The model under review builds one solid part; all positions refer to its coordinate system, in mm. A direction names the side the tool comes from. Round coordinates to 2 decimals unless told otherwise and drop trailing zeros. Order: outer loops, then holes, each group sorted by start corner. A loop starts at its lowest first (then second) coordinate and runs counter-clockwise, first axis right, second up.
1) Machinability: for faces 5 (the face through (0.8, -1.82, -0.54)), 6 (the face through (-0.13, 7.49, 3.79)), 7 (the face through (0, 3, 7.25)), which of the approach directions +Z, -Z, +X, -X, +Y, -Y give a long, thin tool a straight path to every point of the face, cutting with its end or side? Answer none if there is none.
2) Clearance check with flat-ended pins moving along their axes: P1, Ø0.7, axis at x = 0, y = -2, coming from the -Z side; P2, Ø1, axis at x = 3.5, y = -1, coming from the +Z side; P3, Ø3, axis at y = 3.5, z = 2.5, coming from the +X side; P4, Ø0.7, axis at x = 0, y = -2.5, coming from the +Z side. State where each tip first meets the part, or that it passes through.
3) Mouldability with a two-part tool opening along Y and no side actions: class faces 1 (the face through (0, -3.7, -0.6)), 2 (the face through (0, 10.7, 0)), 3 (the face through (-0.694, 3.376, 4.046)), 4 (the face through (-0.8, -1.82, -0.56)) as pulls with the +Y half, pulls with the -Y half, needs draft (parallel to the pull), parting line crosses it, or undercut.
4) To check wall thickness, follow L1, parallel to Y at x = 0, z = 3.75; L2, parallel to Y at x = 2, z = -3.75; L3, parallel to Z at x = 2.25, y = 8. State the ranges of each line that lie inside material, in increasing order.
5) Consider section D-D (x = 1.25). Give the boundary of the cut face in (y, z), then the cut area to 3 significant figures.
6) Consider section B-B (z = 1.25). Give the boundary of the cut face in (x, y).
7) Consider section A-A (y = -1.5). Give the boundary of the cut face in (x, z), then the cut area to 3 significant figures.
8) Consider section C-C (y = 1.75). Give the boundary of the cut face in (x, z), then the cut area to 3 significant figures.
Autodesk Fusion 360 part; units mm, degrees
sketch "Sketch1" plane through (0, 0, 0) normal (0, 1, 0) x (1, 0, 0)
  line L0 (4.5, -7.25) -> (-4.5, -7.25)
  line L1 (-4.5, -7.25) -> (-4.5, 7.25)
  line L2 (-4.5, 7.25) -> (4.5, 7.25)
  line L3 (4.5, 7.25) -> (4.5, -7.25)
  line L4 (4.5, -7.25) -> (-4.5, 7.25) construction
  line L5 (-4.5, -7.25) -> (4.5, 7.25) construction
  line L6 (0, -7.25) -> (0, 7.25) construction
  circle A0 centre (4.8, 3.65) radius 0.5
  circle A1 centre (4.8, 3.05) radius 0.5
  line L7 (4.8, 3.05) -> (5.3, 3.05) construction
  line L8 (4.8, 3.65) -> (5.3, 3.65) construction
  line L9 (5.3, 3.05) -> (5.3, 3.65)
  line L10 (4.8, 3.65) -> (4.3, 3.65) construction
  line L11 (4.8, 3.05) -> (4.3, 3.05) construction
  line L12 (4.3, 3.05) -> (4.3, 3.65)
  line L13 (4.8, 3.05) -> (4.8, 3.65) construction
  line L14 (0.3, 0.05) -> (-0.3, 0.05)
  line L15 (0.3, 0.55) -> (0.3, 1.05) construction
  line L16 (0.3, 0.55) -> (-0.3, 0.55) construction
  line L17 (0.3, 0.55) -> (0.3, 0.05) construction
  line L18 (-0.3, 0.55) -> (-0.3, 0.05) construction
  line L19 (0.3, 1.05) -> (-0.3, 1.05)
  line L20 (-0.3, 0.55) -> (-0.3, 1.05) construction
  circle A2 centre (-0.3, 0.55) radius 0.5
  circle A3 centre (0.3, 0.55) radius 0.5
  line L21 (0.3, 5.85) -> (-0.3, 5.85)
  line L22 (0.3, 6.35) -> (0.3, 6.85) construction
  line L23 (0.3, 6.35) -> (-0.3, 6.35) construction
  line L24 (0.3, 6.35) -> (0.3, 5.85) construction
  line L25 (-0.3, 6.35) -> (-0.3, 5.85) construction
  line L26 (0.3, 6.85) -> (-0.3, 6.85)
  line L27 (-0.3, 6.35) -> (-0.3, 6.85) construction
  circle A4 centre (-0.3, 6.35) radius 0.5
  circle A5 centre (0.3, 6.35) radius 0.5
  point P0 (4.8, 3.35)
  point P1 (0, 0.55)
  point P2 (0, 6.35)
  dimension "d1" = 14.5
  dimension "d2" = 9
  dimension "d19" = 1
  dimension "d20" = 1
  dimension "d21" = 0.6
  dimension "d22" = 10.6
  dimension "d23" = 4.8
  dimension "d24" = 1
  dimension "d25" = 1
  dimension "d27" = 1
  dimension "d28" = 1
  dimension "d30" = 7.8
  dimension "d31" = 13.6
  dimension "d32" = 0.6
  dimension "d33" = 0.6
extrude "Extrude1" add sketch "Sketch1" along normal blind 10.7 contours L0 L1 L2 L3 A0 A1 L12 | L3 A0 A1 | L3 A0 A1 | A0 A1 L12 | L3 A0 A1 | A2 A3 | L14 A2 A3 | A2 A3 | A2 A3 | L19 A2 A3 | A4 A5 | L21 A4 A5 | A4 A5 | A4 A5 | L26 A4 A5 picked at (4.4833, 2.8644) picked at (4.4879, 3.3733) picked at (4.4833, 3.8356) makes body 1
fillet "Fillet1" radius 0.5 8 edges at (4.5, 10.7, 0) (-4.5, 10.7, 0) (-4.5, 0, 0) (4.5, 0, 0) (0, 0, 7.25) (0, 0, -7.25) (0, 10.7, 7.25) (0, 10.7, -7.25) on bodies 1
sketch "Sketch2" plane through (0, 0, 7.25) normal (0, 0, 1) x (1, 0, 0)
  line L0 (-4.5, 0.5) -> (4.5, 0.5)
  line L1 (4.5, 0.5) -> (4.5, 10.2)
  line L2 (4.5, 10.2) -> (-4.5, 10.2)
  line L3 (-4.5, 10.2) -> (-4.5, 0.5)
  line L4 (4.5, 0.5) -> (-4.5, 0.5) construction
  arc A0 (-4.5, 0.5) -> (-4, 0) centre (-4, 0.5) ccw construction
  line L5 (-4, 0) -> (4, 0) construction
  arc A1 (4, 0) -> (4.5, 0.5) centre (4, 0.5) ccw construction
  line L6 (-4.5, 10.2) -> (4.5, 10.2) construction
  arc A2 (4.5, 10.2) -> (4, 10.7) centre (4, 10.2) ccw construction
  line L7 (4, 10.7) -> (-4, 10.7) construction
  arc A3 (-4, 10.7) -> (-4.5, 10.2) centre (-4, 10.2) ccw construction
  line L8 (0, 0) -> (0, 10.7) construction
  circle A4 centre (0, 6.5) radius 1
  circle A5 centre (0, 6.5) radius 3.2
  dimension "d7" = 6.4
  dimension "d8" = 2
  dimension "d9" = 6.5
extrude "Extrude2" cut sketch "Sketch2" against normal blind 6.5 contours A5 bodies 1
fillet "Fillet2" radius 0.5 1 edges at (-0.9323, 6.1384, 7.25) on bodies 1
extrude "Extrude3" add sketch "Sketch1" against normal blind 3.7 contours L3 A0 A1 | L3 A0 A1 | L3 A0 A1 | L3 A0 A1 | A0 A1 L12 | A0 A1 L9 | L3 A0 A1 | L3 A0 A1 | A2 A3 | L14 A2 A3 | A2 A3 | A2 A3 | L19 A2 A3 | A4 A5 | L21 A4 A5 | A4 A5 | A4 A5 | L26 A4 A5 bodies 1 makes body 2 at (5.1986, -1.2333, -3.9519)
extrude "Extrude4" add sketch "Sketch1" along normal blind 4 contours L3 A0 A1 | L3 A0 A1 | L3 A0 A1 | L3 A0 A1 | A0 A1 L12 | A0 A1 L9 | L3 A0 A1 | L3 A0 A1 bodies 1 2
fillet "Fillet3" radius 0.25 3 edges at (5.0236, 4, -2.6028) (5.3, 4, -3.35) (5.0236, 4, -4.0972) on bodies 1
Answer below:
1. face 5: +X, -Y
1. face 6: +Z
1. face 7: +Z, +X, -X, +Y, -Y
2. P1: stops at z = -6.85
2. P2: passes through
2. P3: stops at x = 4.5
2. P4: stops at z = -0.05
3. face 1: pulls with the -Y half
3. face 2: pulls with the +Y half
3. face 3: undercut
3. face 4: needs draft
4. L1: y = 0 to 3.3, 5.5 to 7.5, 9.7 to 10.7
4. L2: y = 0 to 10.7
4. L3: z = -7.25 to 0.75
5. outline: (0, -6.75) arc R0.5 ccw to (0.5, -7.25) - (10.2, -7.25) arc R0.5 ccw to (10.7, -6.75) - (10.7, 6.75) arc R0.5 ccw to (10.2, 7.25) - (9.45, 7.25) - (9.45, 0.75) - (3.55, 0.75) - (3.55, 7.25) - (0.5, 7.25) arc R0.5 ccw to (0, 6.75) - close
5. area: 117 mm2
6. outline: (-4.5, 0.5) arc R0.5 ccw to (-4, 0) - (4, 0) arc R0.5 ccw to (4.5, 0.5) - (4.5, 10.2) arc R0.5 ccw to (4, 10.7) - (-4, 10.7) arc R0.5 ccw to (-4.5, 10.2) - close; circle Ø2 at (0, 6.5); hole circle Ø6.4 at (0, 6.5)
7. outline: (-0.3, -6.85) - (0.3, -6.85) arc R0.5 ccw to (0.3, -5.85) - (-0.3, -5.85) arc R0.5 ccw to start; (-0.3, -1.05) - (0.3, -1.05) arc R0.5 ccw to (0.3, -0.05) - (-0.3, -0.05) arc R0.5 ccw to start; (4.3, -3.65) arc R0.5 ccw to (5.3, -3.65) - (5.3, -3.05) arc R0.5 ccw to (4.3, -3.05) - close
7. area: 4.16 mm2
8. outline: (-4.5, -7.25) - (4.5, -7.25) - (4.5, -4.05) arc R0.5 ccw to (5.3, -3.65) - (5.3, -3.05) arc R0.5 ccw to (4.5, -2.65) - (4.5, 7.25) - (-4.5, 7.25) - close
8. area: 132 mm2
